Autodesk Inventor part; units mm, degrees
ref_plane "YZ Plane" through (0, 0, 0) normal (1, 0, 0) x (0, 1, 0)
ref_plane "XZ Plane" through (0, 0, 0) normal (0, 1, 0) x (-1, 0, 0)
ref_plane "XY Plane" through (0, 0, 0) normal (0, 0, 1) x (1, 0, 0)
sketch "Sketch1" plane through (0, 0, 0) normal (0, 0, 1) x (1, 0, 0)
  line L0 (-136.525, 0) -> (-136.525, -269.875)
  line L1 (-136.525, -269.875) -> (136.525, -269.875)
  line L2 (136.525, -269.875) -> (136.525, 0)
  arc A0 (136.525, 0) -> (-136.525, 0) centre (0, 0) ccw
  dimension "d0" = 273.05
  dimension "d1" = 406.4
extrude "Extrusion1" add sketch "Sketch1" along normal blind 9.525
hole "Hole1" at (-82.55, -244.475, 9.525) direction (0, 0, -1) diameter 6.35 depth 25.4 tip angle 118
hole "Hole2" at (82.55, -244.475, 9.525) direction (0, 0, -1) diameter 6.35 depth 25.4 tip angle 118
hole "Hole3" at (-82.55, -107.95, 9.525) direction (0, 0, -1) diameter 6.35 depth 25.4 tip angle 118
hole "Hole4" at (82.55, -107.95, 9.525) direction (0, 0, -1) diameter 6.35 depth 25.4 tip angle 118
hole "Hole5" at (-82.55, 98.425, 9.525) direction (0, 0, -1) diameter 6.35 depth 25.4 tip angle 118
hole "Hole6" at (82.55, 98.425, 9.525) direction (0, 0, -1) diameter 6.35 depth 25.4 tip angle 118
hole "Hole7" at (0, -180.975, 9.525) direction (0, 0, -1) diameter 158.75 depth 25.4 tip angle 118
properties part number "Bottom_Deck"
Geometry: final body of the model. Coordinates: model frame, mm. Round coordinates to 2 decimals unless told otherwise and drop trailing zeros. Write each loop counter-clockwise with the first axis right and the second up, starting at its lowest first coordinate (ties: lowest second). Pieces come first, ordered by that corner, then holes.
Item 1: Mould query, pull axis X, two halves, no side actions, for faces 1 (the face through (-3.002, 136.492, 4.696)), 2 (the face through (-2, -64, 9.525)), 3 (the face through (-3.49, -101.677, 4.696)). Classes: +X half, -X half, draft (parallel to the pull), parting line (faces both ways), or undercut.
Item 2: Pin query (flat end, axial travel): P1, Ø2, axis at y = 34, z = 4.5, coming from the +X side; P2, Ø4, axis at x = -82.55, y = 98.425, coming from the -Z side; P3, Ø1, axis at x = -18, z = 2.5, coming from the +Y side. Return the tip coordinate at first contact, or that it passes through.
Item 3: Section query C-C (y = -220.5). Return loops of the section in (x, z) (3 decimals), plus the area to 3 significant figures.
Item 4: Section query A-A (z = 2.75). Return loops of the section in (x, y) (3 decimals), plus the area to 3 significant figures.
Item 5: Section query D-D (y = 66.5). Return loops of the section in (x, z) (3 decimals).
Item 6: Section query B-B (x = 30). Return loops of the section in (y, z) (3 decimals).
Item 7: Material intervals for L1, parallel to Y at x = 82.55, z = 4.5 (3 decimals); L2, parallel to X at y = -246, z = 0.5 (3 decimals); L3, parallel to X at y = -107.95, z = 6.5 (3 decimals), sorted ascending.
Completed:
1. face 1: parting line
1. face 2: draft
1. face 3: undercut
2. P1: stops at x = 132.48
2. P2: passes through
2. P3: stops at y = 135.4
3. outline: (-136.525, 0) - (-68.834, 0) - (-68.834, 9.525) - (-136.525, 9.525) - close; (68.834, 0) - (136.525, 0) - (136.525, 9.525) - (68.834, 9.525) - close
3. area: 1,290 mm2
4. outline: (-136.525, -269.875) - (136.525, -269.875) - (136.525, 0) arc R136.525 ccw to (-136.525, 0) - close; hole circle Ø6.35 at (-82.55, -244.475); hole circle Ø6.35 at (-82.55, -107.95); hole circle Ø6.35 at (-82.55, 98.425); hole circle Ø158.75 at (0, -180.975); hole circle Ø6.35 at (82.55, -244.475); hole circle Ø6.35 at (82.55, -107.95); hole circle Ø6.35 at (82.55, 98.425)
4. area: 83,000 mm2
5. outline: (-119.234, 0) - (119.234, 0) - (119.234, 9.525) - (-119.234, 9.525) - close
6. outline: (-269.875, 0) - (-254.462, 0) - (-254.462, 9.525) - (-269.875, 9.525) - close; (-107.488, 0) - (133.188, 0) - (133.188, 9.525) - (-107.488, 9.525) - close
7. L1: y = -269.875 to -247.65, -241.3 to -111.125, -104.775 to 95.25, 101.6 to 108.741
7. L2: x = -136.525 to -85.335, -79.765 to -45.521, 45.521 to 79.765, 85.335 to 136.525
7. L3: x = -136.525 to -85.725, -79.375 to -31.109, 31.109 to 79.375, 85.725 to 136.525
